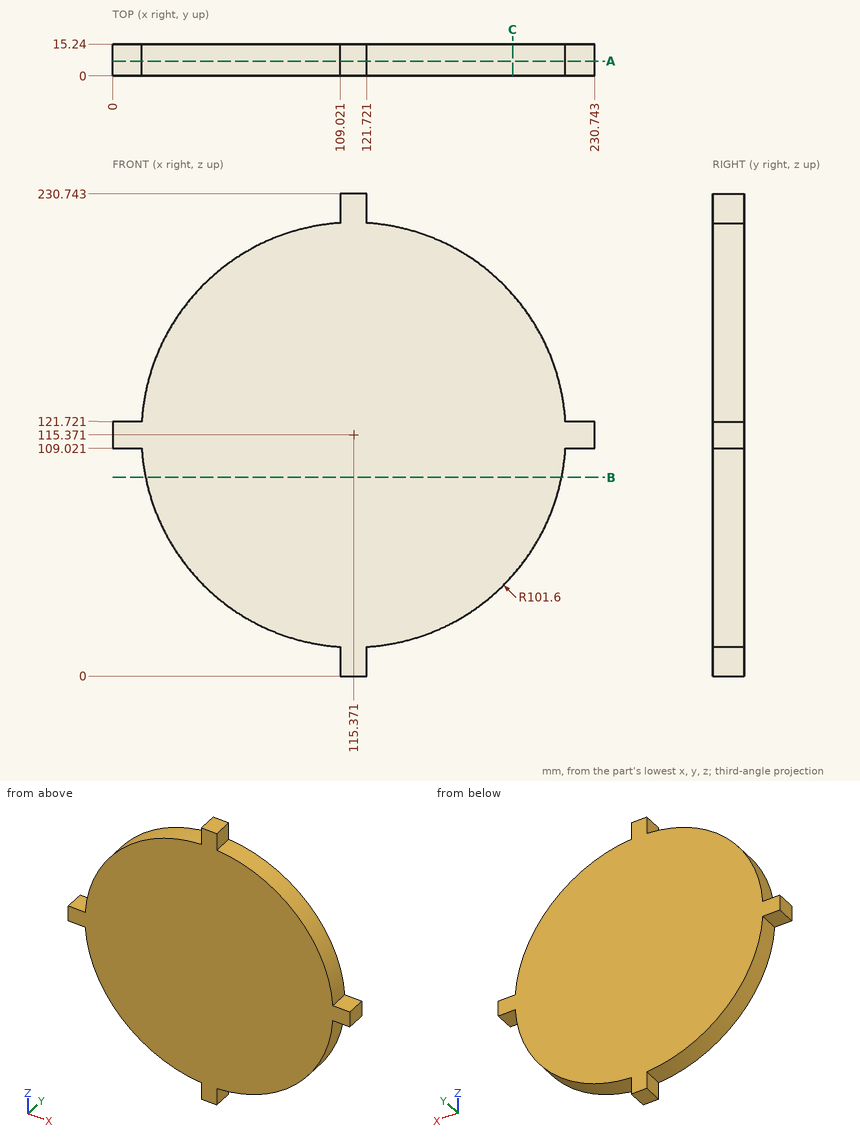
For this review, use the dimensioned drawing (mm, ordinates from the lowest corner) and the shaded views. Give positions to 0.01 mm unless a question says otherwise; leave off trailing zeros. Order: outer loops, then holes, each group sorted by start corner. A loop starts at its lowest first (then second) coordinate and runs counter-clockwise, first axis right, second up. Notation, with made-up numbers: (78.5, 88) - (91.5, 88) arc R19 cw to (91.5, 122) - close; hole circle Ø10 at (4, 71). An arc over 180 degrees is marked (long way). Use CSV: the item, a comma, the result in double quotes. Start each with the question number.
Q1. To check wall thickness, follow line 1 along Z through (x, y) = (12, 8); line 2 along Z through (x, y) = (126, 13.25); line 3 along X through (y, z) = (1.5, 168) (1 decimal). State the ranges of each line that lie inside material, in increasing order. Write a range as [from, to].
Q2. We need section B-B, the plane z = 95. Write out the cut boundary in (x, y) (1 decimal).
Q3. We need section C-C, the plane x = 191.5. Write out the cut boundary in (y, z) (1 decimal).
Q4. Clearance check with flat-ended pins moving along their axes: pin 1 Ø8 at (y, z) = (4.5, 161.5) entering from -X; pin 2 Ø1 at (x, y) = (172.5, 9) entering from +Z; pin 3 Ø4 at (x, y) = (221, 6) entering from -Z. State where each tip first meets the part, or that it passes through.
Q5. We need section A-A, the plane y = 7. Write out the cut boundary in (x, z).
Outcome:
1,line 1,"z = [109.02, 121.72]"
1,line 2,"z = [14.33, 216.41]"
1,line 3,"x = [28.5, 202.3]"
2,outline,"(15.8, 0) - (214.9, 0) - (214.9, 15.2) - (15.8, 15.2) - close"
3,outline,"(0, 48.1) - (15.2, 48.1) - (15.2, 182.7) - (0, 182.7) - close"
4,pin 1,"stops at x = 22.92"
4,pin 2,"stops at z = 199.73"
4,pin 3,"stops at z = 109.02"
5,outline,"(0, 109.02) - (13.97, 109.02) arc R101.6 ccw to (109.02, 13.97) - (109.02, 0) - (121.72, 0) - (121.72, 13.97) arc R101.6 ccw to (216.77, 109.02) - (230.74, 109.02) - (230.74, 121.72) - (216.77, 121.72) arc R101.6 ccw to (121.72, 216.77) - (121.72, 230.74) - (109.02, 230.74) - (109.02, 216.77) arc R101.6 ccw to (13.97, 121.72) - (0, 121.72) - close"
